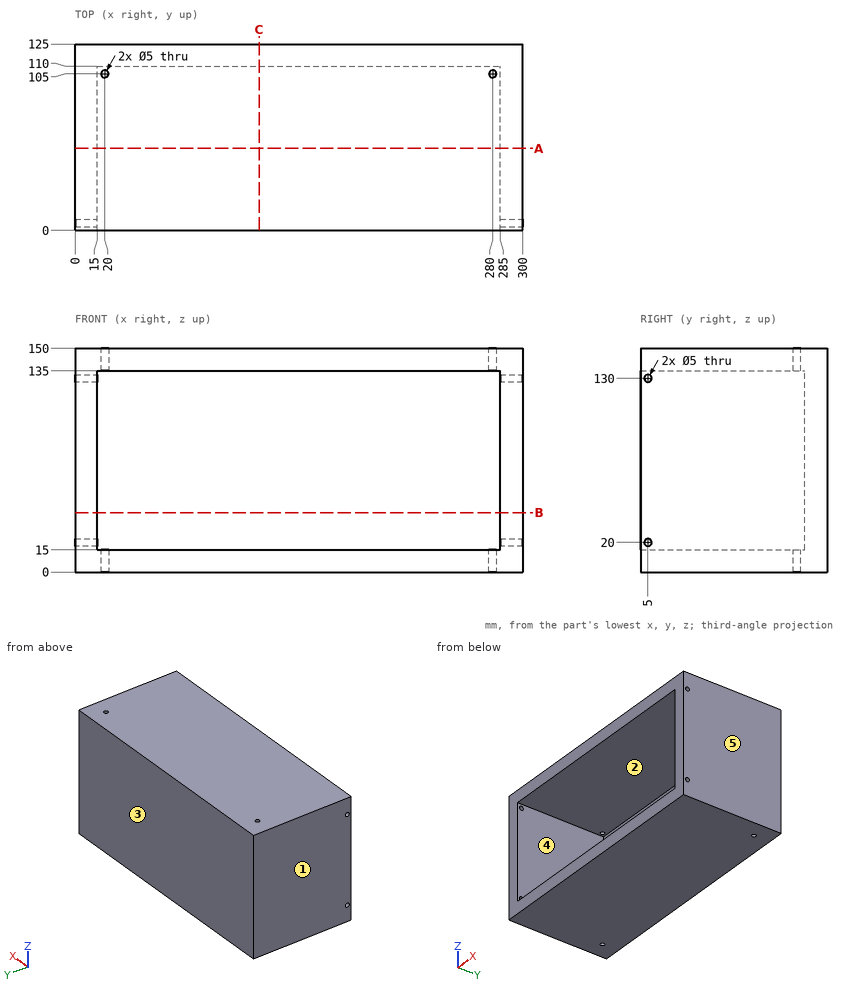
Verification items for this drawing (mm, ordinates from the low corner). A direction names the side the tool comes from. Round coordinates to 2 decimals unless told otherwise and drop trailing zeros. Order: outer loops, then holes, each group sorted by start corner. A loop starts at its lowest first (then second) coordinate and runs counter-clockwise, first axis right, second up. Notation, with made-up numbers: M -20.75,79.5 L 24.25,79.5 A20 cw 24.25,83.5 Z; hole C -1.75,45.5 d8. An arc over 180 degrees is marked long. Answer in a Markdown table with one row per item. Add a question column.
Item 1: Sectioned sample at C-C, the plane x = 123.5. Enter the section's corners in (y, z), plus the area to 3 significant figures.
Item 2: Depth check by flat-ended pin: pin 1 Ø4 at (x, z) = (93, 109) entering from -Y. Enter the tip coordinate at first touch or a pass-through.
Item 3: Set-up check for the marked faces 4 and 5: record each of +Z, -Z, +X, -X, +Y, -Y from which the full face is reachable in a straight line by a thin tool's end or side.
Item 4: Material ranges on L1, parallel to Z at x = 282.5, y = 34; L2, parallel to X at y = 107.5, z = 64; L3, parallel to Y at x = 280, z = 8, recorded low to high. Write a range as [from, to].
Item 5: Sectioned sample at A-A, the plane y = 55. Enter the section's corners in (x, z).
Item 6: Draft check along X on the marked faces 1, 2 and 3. Enter one of: released by +X, released by -X, zero draft, split by the parting line, or undercut.
Item 7: Sectioned sample at B-B, the plane z = 40. Enter the section's corners in (x, y).
Filled in:
| question | item | result |
|---|---|---|
| 1 | outline | M 0,0 L 125,0 L 125,150 L 0,150 L 0,135 L 110,135 L 110,15 L 0,15 Z |
| 1 | area | 5,550 mm² |
| 2 | pin 1 | stops at y = 110 |
| 3 | face 4 | -Y |
| 3 | face 5 | +Z, -Z, +X, +Y, -Y |
| 4 | L1 | z = [0, 15], [135, 150] |
| 4 | L2 | x = [0, 15], [285, 300] |
| 4 | L3 | y = [0, 102.5], [107.5, 125] |
| 5 | outline | M 0,0 L 300,0 L 300,150 L 0,150 Z; hole M 15,15 L 285,15 L 285,135 L 15,135 Z |
| 6 | face 1 | released by -X |
| 6 | face 2 | undercut |
| 6 | face 3 | zero draft |
| 7 | outline | M 0,0 L 15,0 L 15,110 L 285,110 L 285,0 L 300,0 L 300,125 L 0,125 Z |
